```python
from build123d import *

# Parameters (mm, degrees)
F0_W     = 5.2836788818
F0_H     = 2.1386321168
F1_DEPTH = 5.08
F2_R     = 1.9844931554
F3_DEPTH = 20.32


with BuildPart() as f1:
    # F0 (on Front) → F1 (new body)
    with BuildSketch(Plane.XZ):
        with Locations((-15.4736326076, 1.0693160584)):
            Rectangle(F0_W, F0_H)
        Polygon((-12.8317931667, 2.1386321168), (-12.8317931667, 0), (-12.8317931667, -27.8271362185), (-8.6476681754, -27.8271362185), (-8.6476681754, 2.1386321168), align=None)
        Polygon((-18.1154720485, -27.8271362185), (-18.1154720485, 0), (-18.1154720485, 2.1386321168), (-21.9318177551, 2.1386321168), (-21.9318177551, -27.8271362185), align=None)
    extrude(amount=F1_DEPTH)

    # F2 (on face) → F3 (join)
    with BuildSketch(Plane.XY.offset(2.1386321168)):
        with Locations((-15.4426656663, -2.4918615818)):
            Circle(F2_R)
    extrude(amount=F3_DEPTH)


solid = f1.part
```
Geometry check sheet. Reference: the model listing, model coordinates, mm. A direction names the side the tool comes from. Coordinates: 2 decimals unless noted, no trailing zeros. Order: outer loops, then holes, each group sorted by start corner. A loop starts at its lowest first (then second) coordinate and runs counter-clockwise, first axis right, second up. Notation, with made-up numbers: M 69.5,-18.75 L 80.5,-18.75 A16 cw 80.5,12.25 Z; hole C -29,35 d8. An arc over 180 degrees is marked long. Answer as a JSON object with one key per item and string values.
Q1. Cross-section at D-D on z = 3. Record the cut outline in (x, y), and give its area (3 significant figures).
Results are:
{"outline": "C -15.44,-2.49 d3.97", "area": "12.4 mm²"}
Q2. Cross-section at B-B on x = -14.25. Record the cut outline in (y, z), and give its area (3 significant figures).
Results are:
{"outline": "M -5.08,0 L 0,0 L 0,2.14 L -0.91,2.14 L -0.91,22.46 L -4.08,22.46 L -4.08,2.14 L -5.08,2.14 Z", "area": "75.3 mm²"}
Q3. Tool access check on faces 1 (the flat face through (-18.3, 0, -12.6)), 2 (the cylindrical face through (-17.425, -2.405, 12.156)), 3 (the flat face through (-16, -3, 0)). Record the directions out of +Z, -Z, +X, -X, +Y, -Y that give a thin tool (end or side, any length) a straight path to the whole face; none if there is none.
Results are:
{"face 1": "+Z, -Z, +X, -X, +Y", "face 2": "+Z", "face 3": "-Z, +Y, -Y"}
Q4. Cross-section at A-A on z = -18. Record the cut outline in (x, y).
Results are:
{"outline": "M -21.93,-5.08 L -18.12,-5.08 L -18.12,0 L -21.93,0 Z; M -12.83,-5.08 L -8.65,-5.08 L -8.65,0 L -12.83,0 Z"}
Q5. Depth check by flat-ended pin: pin 1 Ø2 at (x, z) = (-18, 12.5) entering from -Y; pin 2 Ø1.5 at (x, y) = (-15, -4) entering from -Z. Enter the tip coordinate at first touch or a pass-through.
Results are:
{"pin 1": "stops at y = -3.72", "pin 2": "stops at z = 0"}
Q6. Cross-section at C-C on y = -3.6. Record the cut outline in (x, z).
Results are:
{"outline": "M -21.93,-27.83 L -18.12,-27.83 L -18.12,0 L -12.83,0 L -12.83,-27.83 L -8.65,-27.83 L -8.65,2.14 L -13.8,2.14 L -13.8,22.46 L -17.09,22.46 L -17.09,2.14 L -21.93,2.14 Z"}
Q7. Scan lines: line 1 (X direction, y = -0.95, z = -16); line 2 (Z direction, x = -12, y = -3.95); line 3 (Z direction, x = -16, y = -0.75). Record each from-to range of solid material in increasing order.
Results are:
{"line 1": "x = -21.93 to -18.12, -12.83 to -8.65", "line 2": "z = -27.83 to 2.14", "line 3": "z = 0 to 22.46"}
